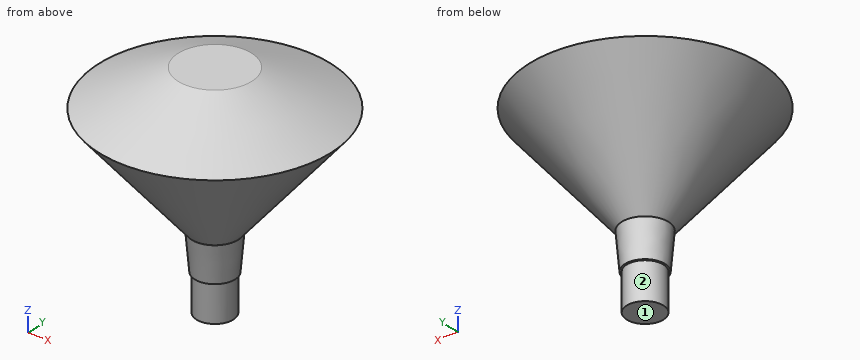
```python
from build123d import *

# Parameters (mm, degrees)
F0_R     = 12.7
F1_DEPTH = 25.4
F2_R     = 13.889054696
F3_DEPTH = 25.4
F3_TAPER = -5
F4_R     = 16.0431717149
F5_DEPTH = 76.2
F5_TAPER = -40
F6_R     = 79.7788549735
F7_DEPTH = 25.4
F7_TAPER = 65


with BuildPart() as f1:
    # F0 (on Top) → F1 (new body)
    with BuildSketch(Plane.XY):
        Circle(F0_R)
    extrude(amount=F1_DEPTH)

    # F2 (on face) → F3 (join)
    with BuildSketch(Plane.XY.offset(25.4)):
        Circle(F2_R)
    extrude(amount=F3_DEPTH, taper=F3_TAPER)

    # F4 (on face) → F5 (join)
    with BuildSketch(Plane.XY.offset(50.8)):
        Circle(F4_R)
    extrude(amount=F5_DEPTH, taper=F5_TAPER)

    # F6 (on face) → F7 (join)
    with BuildSketch(Plane.XY.offset(127)):
        Circle(F6_R)
    extrude(amount=F7_DEPTH, taper=F7_TAPER)


solid = f1.part
```
Geometry: final body of the model. Coordinates: model frame, mm. Face numbers are marked on the shaded views. A direction names the side the tool comes from. Round coordinates to 2 decimals unless told otherwise and drop trailing zeros. Write each loop counter-clockwise with the first axis right and the second up, starting at its lowest first coordinate (ties: lowest second). Pieces come first, ordered by that corner, then holes. Notation, with made-up numbers: M 50,38.5 L 71,38.5 A14 ccw 71,44.5 Z; hole C -13,85 d10. An arc over 180 degrees is marked long. Answer in a Markdown table with one row per item. Add a question column.
(1) Reachability of the marked faces 1 and 2 from +Z, -Z, +X, -X, +Y, -Y: full face, straight path, thin tool, end or side. Return the list, or none.
(2) Cut plane B-B, the plane x = 0. Return the cut outline in (y, z), then the cut area to 3 significant figures.
(3) Cut plane C-C, the plane z = 119.5. Return the cut outline in (x, y).
(4) Cut plane A-A, the plane z = 13.5. Return the cut outline in (x, y), then the cut area to 3 significant figures.
(5) Contact query for flat-ended pins moving along their axis: pin 1 (8 mm diameter, centred on x = 36.5, y = 48.5, fed in from +Z); pin 2 (1 mm diameter, centred on x = -40, y = -17.5, fed in from +Z); pin 3 (12 mm diameter, centred on y = -26, z = 53, fed in from -X); pin 4 (1.5 mm diameter, centred on x = -9.5, z = 63, fed in from -Y). Output: stop coordinate, or through.
(6) Ray query, L1, parallel to X at y = 13, z = 116; L2, parallel to Z at x = -62, y = 8.5; L3, parallel to X at y = -21, z = 97. Return the intervals inside material, ascending.
Established:
| question | item | result |
|---|---|---|
| 1 | face 1 | -Z, +X, -X, +Y, -Y |
| 1 | face 2 | -Z |
| 2 | outline | M -79.98,127 L -16.04,50.8 L -16.11,50.8 L -13.89,25.4 L -12.7,25.4 L -12.7,0 L 12.7,0 L 12.7,25.4 L 13.89,25.4 L 16.11,50.8 L 16.04,50.8 L 79.98,127 L 79.78,127 L 25.31,152.4 L -25.31,152.4 L -79.78,127 Z |
| 2 | area | 11,400 mm² |
| 3 | outline | C 0,0 d147.38 |
| 4 | outline | C 0,0 d25.4 |
| 4 | area | 507 mm² |
| 5 | pin 1 | z = 137.76 |
| 5 | pin 2 | z = 144.08 |
| 5 | pin 3 | through |
| 5 | pin 4 | y = -25.23 |
| 6 | L1 | -69.55 to 69.55 |
| 6 | L2 | 106.26 to 135.02 |
| 6 | L3 | -50.63 to 50.63 |
